Read the model definition and answer for the solid it produces. Units are mm, in the model's axes. Face numbers are marked on the shaded views. A direction names the side the tool comes from. Coordinates: 2 decimals unless noted, no trailing zeros. Write each loop counter-clockwise with the first axis right and the second up, starting at its lowest first coordinate (ties: lowest second). Pieces come first, ordered by that corner, then holes.
(1) Section C-C on y = 54.5 is taken. Write down the section's boundary in (x, z).
(2) Section D-D on z = -4.5 is taken. Write down the section's boundary in (x, y), then the cut area to 3 significant figures.
(3) Given pin 1 (9 mm diameter, centred on y = 28.5, z = -32, fed in from +X); pin 2 (9 mm diameter, centred on x = 25, y = 45.5, fed in from -Z), each flat-ended and moving along its own axis, determine where each tip first touches the part or whether it passes through.
(4) Section A-A on z = -30 is taken. Write down the section's boundary in (x, y), then the cut area to 3 significant figures.
(5) Section B-B on x = 18 is taken. Write down the section's boundary in (y, z), then the cut area to 3 significant figures.
(6) Find the intervals of material crossed by probe 1 along X at (y, z) = (52, -22); probe 2 along Z at (x, y) = (11, 42); probe 3 along Z at (x, y) = (3, 12), in increasing order.
(7) Which of the six approach directions +Z, -Z, +X, -X, +Y, -Y give full straight-line access (tool end or side, diameter ignored) to the marked faces 1 and 2?
from build123d import *

# Parameters (mm, degrees)
BOSS_EXTRUDE1_DEPTH = 80
FILLET1_R           = 7.5


with BuildPart() as part:
    # Sketch1 → Boss-Extrude1 (new body)
    with BuildSketch(Plane(origin=(0, 0, 0), x_dir=(1, 0, 0), z_dir=(0, 1, 0))):
        Polygon((40, 6.65), (10, 6.65), (10, 3.35), (40, 3.35), (40, 0), (0, 0), (0, 40), (3.35, 40), (3.35, 10), (6.65, 10), (6.65, 40), (10, 40), (10, 10), (40, 10), align=None)
    extrude(amount=BOSS_EXTRUDE1_DEPTH)

    # Fillet1
    fillet1_edges = [part.edges().sort_by_distance(p)[0] for p in [
        (0, 40, 0),
    ]]
    fillet(fillet1_edges, radius=FILLET1_R)


solid = part.part
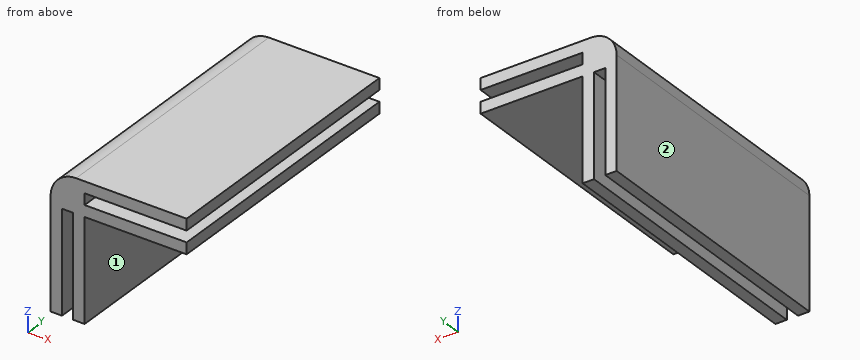
Response:
1. outline: (0, -40) - (3.35, -40) - (3.35, -10) - (6.65, -10) - (6.65, -40) - (10, -40) - (10, -10) - (40, -10) - (40, -6.65) - (10, -6.65) - (10, -3.35) - (40, -3.35) - (40, 0) - (7.5, 0) arc R7.5 ccw to (0, -7.5) - close
2. outline: (0.63, 0) - (10, 0) - (10, 80) - (0.63, 80) - close
2. area: 750 mm2
3. pin 1: stops at x = 10
3. pin 2: stops at z = -10
4. outline: (0, 0) - (3.35, 0) - (3.35, 80) - (0, 80) - close; (6.65, 0) - (10, 0) - (10, 80) - (6.65, 80) - close
4. area: 536 mm2
5. outline: (0, -10) - (80, -10) - (80, -6.65) - (0, -6.65) - close; (0, -3.35) - (80, -3.35) - (80, 0) - (0, 0) - close
5. area: 536 mm2
6. probe 1: x = 0 to 3.35, 6.65 to 10
6. probe 2: z = -10 to -6.65, -3.35 to 0
6. probe 3: z = -40 to -1.5
7. face 1: -Z, +X, +Y, -Y
7. face 2: +Z, -Z, -X, +Y, -Y
